```python
from build123d import *

# Parameters (mm, degrees)
BOSS_EXTRUDE1_DEPTH   = 15
BOSS_EXTRUDE2_DEPTH   = 10
BOSS_EXTRUDE2_2_DEPTH = 10
BOSS_EXTRUDE3_DEPTH   = 1
BOSS_EXTRUDE8_DEPTH   = 2


with BuildPart() as part:
    # Sketch1 → Boss-Extrude1 (new, symmetric)
    with BuildSketch(Plane.XY):
        with BuildLine():
            Line((-30, 0), (-20, 0))
            ThreePointArc((-20, 0), (0, 20), (20, 0))
            Line((20, 0), (30, 0))
            ThreePointArc((30, 0), (0, 30), (-30, 0))
        make_face()
    extrude(amount=BOSS_EXTRUDE1_DEPTH, both=True)



with BuildPart() as body_2:
    # Sketch1<3> → Boss-Extrude2 (new, symmetric)
    with BuildSketch(Plane.XY):
        with BuildLine():
            Line((-130, 0), (-125, 0))
            ThreePointArc((-125, 0), (-110, 15), (-95, 0))
            Line((-95, 0), (-90, 0))
            ThreePointArc((-90, 0), (-110, 20), (-130, 0))
        make_face()
    extrude(amount=BOSS_EXTRUDE2_DEPTH, both=True)


with BuildPart() as body_3:
    # Sketch1<3> → Boss-Extrude2 2 (new, symmetric)
    with BuildSketch(Plane.XY):
        with BuildLine():
            Line((90, 0), (95, 0))
            ThreePointArc((95, 0), (110, 15), (125, 0))
            Line((125, 0), (130, 0))
            ThreePointArc((130, 0), (110, 20), (90, 0))
        make_face()
    extrude(amount=BOSS_EXTRUDE2_2_DEPTH, both=True)


with BuildPart() as part_1:
    add(part.part)

    add(body_2.part)  # Boss-Extrude3 merges body 2

    add(body_3.part)  # Boss-Extrude3 merges body 3
    # Sketch2 → Boss-Extrude3 (add, symmetric)
    with BuildSketch(Plane.XY):
        with BuildLine():
            Line((-111.818181818, 19.917183909), (-2.727272727, 29.875775864))
            ThreePointArc((-2.727272727, 29.875775864), (-22.156468376, 20.225995874), (-30, 0))
            Line((-30, 0), (-90, 0))
            ThreePointArc((-90, 0), (-96.516002751, 14.770978918), (-111.818181818, 19.917183909))
        make_face()
        with BuildLine():
            Line((2.727272727, 29.875775864), (111.818181818, 19.917183909))
            ThreePointArc((111.818181818, 19.917183909), (96.516002751, 14.770978918), (90, 0))
            Line((90, 0), (30, 0))
            ThreePointArc((30, 0), (22.156468376, 20.225995874), (2.727272727, 29.875775864))
        make_face()
    extrude(amount=BOSS_EXTRUDE3_DEPTH, both=True)

    # Sketch3 → Boss-Extrude8 (add)
    with BuildSketch(Plane(origin=(0, 0, 0), x_dir=(1, 0, 0), z_dir=(0, 1, 0))):
        Polygon((91, 10), (91, -10), (29.5, -15), (29.5, 15), align=None)
        Polygon((-29.5, 15), (-29.5, -15), (-91, -10), (-91, 10), align=None)
    extrude(amount=BOSS_EXTRUDE8_DEPTH)


solid = part_1.part
```
The listing builds one solid part. Answer for the finished solid, in the listing's coordinates (mm). A direction names the side the tool comes from. Give positions to 0.01 mm unless a question says otherwise; leave off trailing zeros. Order: outer loops, then holes, each group sorted by start corner. A loop starts at its lowest first (then second) coordinate and runs counter-clockwise, first axis right, second up. Notation, with made-up numbers: (-24.75, 33.5) - (9.25, 33.5) arc R18 ccw to (9.25, 65.5) - close; hole circle Ø10 at (49.25, -24.5). An arc over 180 degrees is marked (long way). Answer in a Markdown table with one row per item. Add a question column.
Q1. The part is cut by section D-D (x = 0). Determine the outline of the cut face in (y, z).
Q2. For a pull along X with two mould halves and no side action, classify faces 1 (the flat face through (127, 0, 0)), 2 (the flat face through (60.039, 0.986, -12.517)), 3 (the cylindrical face through (0.66, 29.993, 0.21)), 4 (the flat face through (-60, 2, 6)) as released by +X, released by -X, zero draft, split by the parting line, or undercut.
Q3. The part is cut by section A-A (y = 5). Give the number of separate pieces and of enclosed holes in the cut face, then the cut area to 3 significant figures.
Q4. Given P1, Ø12, axis at y = 20.5, z = -9.5, coming from the +X side (3 decimals); P2, Ø11, axis at x = -60, z = 7, coming from the +Y side; P3, Ø6, axis at x = -118.5, y = 12.5, coming from the +Z side; P4, Ø10, axis at x = 28, y = 11.5, coming from the -Z side, each flat-ended and moving along its own axis, determine where each tip first touches the part or whether it passes through.
Q5. The part is cut by section C-C (x = -71). Determine the outline of the cut face in (y, z).
Q6. The part is cut by section B-B (z = 6.5). Determine the outline of the cut face in (x, y).
Q7. Which of the six approach directions +Z, -Z, +X, -X, +Y, -Y give full straight-line access (tool end or side, diameter ignored) to faces 5 (the flat face through (-110, 17, -10)), 6 (the flat face through (0, 22, -15)), 7 (the flat face through (110, 17, -10)), 8 (the flat face through (-57, 13, -1))?
Q8. Find the intervals of material crossed by line 1 along X through (y, z) = (11, 0.5); line 2 along X through (y, z) = (4.5, 8); line 3 along X through (y, z) = (6, 8), in increasing order. Write a range as [from, to].
Determined:
| question | item | result |
|---|---|---|
| 1 | outline | (20, -15) - (30, -15) - (30, 15) - (20, 15) - close |
| 2 | face 1 | zero draft |
| 2 | face 2 | released by +X |
| 2 | face 3 | undercut |
| 2 | face 4 | undercut |
| 3 | separate pieces | 4 |
| 3 | enclosed holes | 0 |
| 3 | area | 1,270 mm² |
| 4 | P1 | stops at x = 123.775 |
| 4 | P2 | stops at y = 2 |
| 4 | P3 | stops at z = 10 |
| 4 | P4 | stops at z = -15 |
| 5 | outline | (0, -11.63) - (2, -11.63) - (2, -1) - (23.64, -1) - (23.64, 1) - (2, 1) - (2, 11.63) - (0, 11.63) - close |
| 6 | outline | (-130, 0) - (-125, 0) arc R15 cw to (-95, 0) - (-20, 0) arc R20 cw to (20, 0) - (95, 0) arc R15 cw to (125, 0) - (130, 0) arc R20 ccw to (90.1, 2) - (29.93, 2) arc R30 ccw to (-29.93, 2) - (-90.1, 2) arc R20 ccw to start |
| 7 | face 5 | -Z, -X, +Y, -Y |
| 7 | face 6 | -Z, +X, -X, +Y, -Y |
| 7 | face 7 | -Z, +X, +Y, -Y |
| 7 | face 8 | -Z, +Y |
| 8 | line 1 | x = [-126.7, -120.2], [-99.8, -16.7], [16.7, 99.8], [120.2, 126.7] |
| 8 | line 2 | x = [-129.49, -124.31], [-95.69, -90.51], [-29.66, -19.49], [19.49, 29.66], [90.51, 95.69], [124.31, 129.49] |
| 8 | line 3 | x = [-129.08, -123.75], [-96.25, -90.92], [-29.39, -19.08], [19.08, 29.39], [90.92, 96.25], [123.75, 129.08] |
